from build123d import *

# Parameters (mm, degrees)
SKETCH_7_R = 0.75


with BuildPart() as part:
    # По траектории9: sweep along a path in Эскиз1
    with BuildLine(Plane(origin=(0, 0, 0), x_dir=(1, 0, 0), z_dir=(0, 1, 0))) as sweep_9_path:
        Line((-2.921672053, 0.326690485), (-2.921672053, 15.31971545))
        ThreePointArc((-2.921672053, 15.31971545), (-2.335885615, 16.733929012), (-0.921672053, 17.31971545))
        Line((-0.921672053, 17.31971545), (2.398327947, 17.31971545))
        ThreePointArc((2.398327947, 17.31971545), (3.812541509, 16.733929012), (4.398327947, 15.31971545))
        Line((4.398327947, 15.31971545), (4.398327947, 0.326690485))
    # Эскиз7 → По траектории9 (sweep)
    with BuildSketch(Plane(origin=(-2.921672053, 0, -0.326690485), x_dir=(-1, 0, 0), z_dir=(0, 0, -1))):
        Circle(SKETCH_7_R)
    sweep(path=sweep_9_path.line)


solid = part.part
Check sheet for the modelled part. Datum: model origin and axes. Units: mm. A direction names the side the tool comes from. Give positions to 0.01 mm unless a question says otherwise; leave off trailing zeros. Write each loop counter-clockwise with the first axis right and the second up, starting at its lowest first coordinate (ties: lowest second). Pieces come first, ordered by that corner, then holes. Notation, with made-up numbers: (-36, 7) -> (-15, 7) arc R19 cw to (-15, 34) -> close; hole circle Ø4 at (13, 70.25). An arc over 180 degrees is marked (long way). Use one line per item in the form item = value. Start each with the question number.
1. Section check C-C (x = -0.5). Record the cut outline in (y, z).
2. Thickness scan on line 1 along X through (y, z) = (-0.05, -6); line 2 along X through (y, z) = (0.3, -15); line 3 along Y through (x, z) = (-3.5, -1.5). Record the ranges inside material, lowest first. Write a range as from..to.
3. Access from +Z, -Z, +X, -X, +Y, -Y to the whole of each face (thin tool, end or side, straight path). Record for faces 3 (the cylindrical face through (3.65, 0.03, -7.72)), 4 (the flat face through (-3, 0, -0.327)), 5 (the cylindrical face through (0.762, 0.225, -18.035)).
4. Section check A-A (y = 0). Record the cut outline in (x, z), and give its area (3 significant figures).
5. Section check B-B (z = -14.5). Record the cut outline in (x, y), and give its area (3 significant figures).
6. Mould release check, pull along X, two halves, no side actions. Record for faces 1 (the flat face through (4, 0, -0.327)), 2 (the cylindrical face through (-2.33, -0.46, -7.93)): pulls with the +X half, pulls with the -X half, needs draft (parallel to the pull), parting line crosses it, or undercut.
Conclusion:
q1.outline = circle Ø1.5 at (0, -17.32)
q2.line_1 = -3.67..-2.17, 3.65..5.15
q2.line_2 = -3.61..-2.23, 3.71..5.09
q2.line_3 = -0.48..0.48
q3.face_3 = +Z
q3.face_4 = +Z, +X, -X, +Y, -Y
q3.face_5 = none
q4.outline = (-3.67, -15.32) arc R2.75 ccw to (-0.92, -18.07) -> (2.4, -18.07) arc R2.75 ccw to (5.15, -15.32) -> (5.15, -0.33) -> (3.65, -0.33) -> (3.65, -15.32) arc R1.25 cw to (2.4, -16.57) -> (-0.92, -16.57) arc R1.25 cw to (-2.17, -15.32) -> (-2.17, -0.33) -> (-3.67, -0.33) -> close
q4.area = 59.4 mm²
q5.outline = circle Ø1.5 at (-2.92, 0); circle Ø1.5 at (4.4, 0)
q5.area = 3.53 mm²
q6.face_1 = needs draft
q6.face_2 = undercut
